For this review, take the finished solid that the model builds, in its own axes (mm). A direction names the side the tool comes from. Coordinates: 2 decimals unless noted, no trailing zeros. Order: outer loops, then holes, each group sorted by start corner. A loop starts at its lowest first (then second) coordinate and runs counter-clockwise, first axis right, second up.
from build123d import *

# Parameters (mm, degrees)
ESQUISSE1_R        = 5
BOSS_EXTRU_1_DEPTH = 60
ESQUISSE2_R        = 5
BOSS_EXTRU_2_DEPTH = 20
COQUE1_START       = -1e-07
COQUE1_OUTLINE_R   = 3
COQUE1_DEPTH       = 20.0000001
COQUE1_2_OUTLINE_R = 3
COQUE1_2_DEPTH     = 60


with BuildPart() as part:
    # Esquisse1 → Boss.-Extru.1 (new body)
    with BuildSketch(Plane.XY):
        Circle(ESQUISSE1_R)
    extrude(amount=BOSS_EXTRU_1_DEPTH)

    # Esquisse2 → Boss.-Extru.2 (add)
    with BuildSketch(Plane(origin=(0, 0, 0), x_dir=(0, 0, -1), z_dir=(1, 0, 0))):
        with Locations((-15, 0)):
            Circle(ESQUISSE2_R)
        with Locations((-30, 0)):
            Circle(ESQUISSE2_R)
        with Locations((-45, 0)):
            Circle(ESQUISSE2_R)
    extrude(amount=BOSS_EXTRU_2_DEPTH)

    # Coque1: read off the stored shape, not the designer's step
    # Coque1 outline → Coque1 (cut)
    with BuildSketch(Plane.YZ.offset(COQUE1_START)):
        with Locations((0, 15)):
            Circle(COQUE1_OUTLINE_R)
        with Locations((0, 30)):
            Circle(COQUE1_OUTLINE_R)
        with Locations((0, 45)):
            Circle(COQUE1_OUTLINE_R)
    extrude(amount=COQUE1_DEPTH, mode=Mode.SUBTRACT)

    # Coque1 2 outline → Coque1 2 (cut)
    with BuildSketch(Plane.XY):
        Circle(COQUE1_2_OUTLINE_R)
    extrude(amount=COQUE1_2_DEPTH, mode=Mode.SUBTRACT)


solid = part.part
1. To check wall thickness, follow L1, parallel to Z at x = 7.25, y = 0; L2, parallel to Z at x = 10.75, y = -3.75; L3, parallel to Z at x = 3.75, y = -1.75. State the ranges of each line that lie inside material, in increasing order.
Answer below:
L1: z = 10 to 12, 18 to 20, 25 to 27, 33 to 35, 40 to 42, 48 to 50
L2: z = 11.69 to 18.31, 26.69 to 33.31, 41.69 to 48.31
L3: z = 0 to 12.56, 17.44 to 27.56, 32.44 to 42.56, 47.44 to 60
2. Take a section at A-A, the plane x = 9.25. Give the boundary of the cut face in (y, z).
Answer below:
outline: circle Ø10 at (0, 15); circle Ø10 at (0, 30); circle Ø10 at (0, 45); hole circle Ø6 at (0, 15); hole circle Ø6 at (0, 30); hole circle Ø6 at (0, 45)
3. Clearance check with flat-ended pins moving along their axes: pin 1 Ø1 at (y, z) = (-3.5, 32) entering from -X; pin 2 Ø2 at (x, z) = (17, 11.5) entering from -Y; pin 3 Ø3 at (y, z) = (2, 51.5) entering from -X; pin 4 Ø5.5 at (x, y) = (0, 0) entering from -Z. State where each tip first meets the part, or that it passes through.
Answer below:
pin 1: stops at x = -4
pin 2: stops at y = -4.33
pin 3: stops at x = -4.97
pin 4: passes through
4. Take a section at B-B, the plane y = 0. Give the number of separate pieces and of enclosed holes in the cut face, plus the area to 3 significant figures.
Answer below:
separate pieces: 5
enclosed holes: 0
area: 384 mm2
5. Take a section at C-C, the plane z = 30. Give the boundary of the cut face in (x, y).
Answer below:
outline: (0, -5) - (20, -5) - (20, -3) - (0, -3) arc R3 cw to (0, 3) - (20, 3) - (20, 5) - (0, 5) arc R5 ccw to start
6. The part is to be moulded in two halves that separate along Z. For faces 4 (the face through (-0.1, -3.3, 0)), 5 (the face through (10, 0, 48)), 6 (the face through (-0.1, -3.3, 60)), say which applies: +Z half, -Z half, draft (parallel to the pull), parting line (faces both ways), or undercut.
Answer below:
face 4: -Z half
face 5: undercut
face 6: +Z half
7. Machinability: for faces 1 (the face through (12, 4, 27)), 2 (the face through (-5, 0, 30)), 3 (the face through (20, -3.3, 30.1)), which of the approach directions +Z, -Z, +X, -X, +Y, -Y give a long, thin tool a straight path to every point of the face, cutting with its end or side? Answer none if there is none.
Answer below:
face 1: +X
face 2: none
face 3: +Z, -Z, +X, +Y, -Y
